from build123d import *

# Parameters (mm, degrees)
F0_R        = 1.5875
F1_DEPTH    = 6.35
F2_R        = 10.795
F4_R        = 19.05
F6_T        = 3.175
F6_T3_DEPTH = 12.7
F7_R        = 6.477
F8_DEPTH    = 19.051
F9_R        = 5.08


# Not quite as in the source:
# - two fillets or chamfers of one size are made in one step
# - a shell that OpenCascade refuses in one call is made with other operations: the cavity is built on its own and cut out


with BuildPart() as f1:
    # F0 (on Front) → F1 (new body)
    with BuildSketch(Plane.XZ):
        with BuildLine():
            ThreePointArc((35.2153805779, 11.4421707601), (39.8917386836, 9.0594472943), (42.2744621493, 13.7358054))
            ThreePointArc((42.2744621493, 13.7358054), (0, 44.45), (-42.2744621493, 13.7358054))
            ThreePointArc((-42.2744621493, 13.7358054), (-39.8917386836, 9.0594472943), (-35.2153805779, 11.4421707601))
            ThreePointArc((-35.2153805779, 11.4421707601), (-18.0952762982, 14.4949657749), (-6.0392088785, 1.9622579143))
            ThreePointArc((-6.0392088785, 1.9622579143), (0, -6.35), (6.0392088785, 1.9622579143))
            ThreePointArc((6.0392088785, 1.9622579143), (18.0952762982, 14.4949657749), (35.2153805779, 11.4421707601))
        make_face()
        Circle(F0_R, mode=Mode.SUBTRACT)
        with Locations((-39.2548577101, 12.7546764428)):
            Circle(F0_R, mode=Mode.SUBTRACT)
        with Locations((39.2548577101, 12.7546764428)):
            Circle(F0_R, mode=Mode.SUBTRACT)
        with Locations((-12.7546764428, 39.2548577101)):
            Circle(F0_R, mode=Mode.SUBTRACT)
        with Locations((12.7546764428, 39.2548577101)):
            Circle(F0_R, mode=Mode.SUBTRACT)
    extrude(amount=F1_DEPTH)

    # F2 (on face) → F5 section 0
    with BuildSketch(Plane.XZ.offset(6.35)):
        with Locations((0, 28.575)):
            Circle(F2_R)
    # F4 (on offset) → F5 section 1
    with BuildSketch(Plane.XZ.offset(19.05)):
        with Locations((0, 28.575)):
            Circle(F4_R)
    loft()

    # F6: shell of thickness 3.175, made by hand


with BuildPart() as f6_core1:
    # F6_t2: copy of F1
    add(f1.part)

    # the walls: a layer under each face that stays
    f6_faces = [f6_core1.faces().sort_by_distance(p)[0] for p in [
        (18.0952762982, -3.175, 14.4949657749),
        (0, -3.175, -6.35),
        (39.8917386836, -3.175, 9.0594472943),
        (0, 0, 19.05),
        (-28.3040667791, -6.35, 19.05),
        (-18.0952762982, -3.175, 14.4949657749),
        (0, -3.175, 44.45),
        (-39.8917386836, -3.175, 9.0594472943),
        (-1.5875, -3.175, 0),
        (-40.8423577101, -3.175, 12.7546764428),
        (37.6673577101, -3.175, 12.7546764428),
        (-14.3421764428, -3.175, 39.2548577101),
        (11.1671764428, -3.175, 39.2548577101),
        (-14.9225, -12.7, 28.575),
    ]]
    thicken(f6_faces, amount=-F6_T, mode=Mode.SUBTRACT)

    # F6_s4 → F6_t3 (cut)
    with BuildSketch(Plane.XZ.offset(-3.175)):
        Polygon((6.0999585135, 1.9634355139), (2.9838498192, 2.8256269079), (2.7217112336, 1.8979499721), (3.0196044392, 0.9811289571), align=None)
        Polygon((35.1655409151, 11.4074157187), (37.179742419, 13.9365459438), (37.9370918115, 13.3401207322), (38.2349850172, 12.4232997172), align=None)
        Polygon((-6.0999585135, 1.9634355139), (-3.0196044392, 0.9811289571), (-2.7217112336, 1.8979499721), (-2.9838498192, 2.8256269079), align=None)
        Polygon((-35.1655409151, 11.4074157187), (-37.179742419, 13.9365459438), (-37.9370918115, 13.3401207322), (-38.2349850172, 12.4232997172), align=None)
    extrude(amount=F6_T3_DEPTH, mode=Mode.SUBTRACT)

    # F6_s5 → F6_t6 (revolve, cut)
    with BuildSketch(Plane.XY.offset(28.575)):
        Polygon((10.8216205848, -6.3644466199), (10.795, -3.175), (4.9444718097, -3.175), (8.1329415182, -8.0803380131), align=None)
    revolve(axis=Axis((0, -6.35, 28.575), (0, -1, 0)), mode=Mode.SUBTRACT)


with BuildPart() as f1_1:
    add(f1.part)

    # what is left inside the walls is the cavity
    f6_cavity = [f6_core1.part.solids().sort_by_distance(p)[0] for p in [
        (-10.483081, -11.754195, 28.575),
    ]]
    add(f6_cavity, mode=Mode.SUBTRACT)

    # F7 (on face) → F8 (cut, through all)
    with BuildSketch(Plane.XZ.offset(19.05)):
        with Locations((0, 28.575)):
            Circle(F7_R)
    extrude(amount=-F8_DEPTH, mode=Mode.SUBTRACT)

    # F9
    f9_edges = [f1_1.edges().sort_by_distance(p)[0] for p in [
        (6.039209, -3.175, 1.962258),
        (-6.039209, -3.175, 1.962258),
        (-15.263222, -19.05, 28.575),
    ]]
    fillet(f9_edges, radius=F9_R)


solid = f1_1.part
Check sheet for the modelled part. Datum: model origin and axes. Units: mm. A direction names the side the tool comes from. Round coordinates to 2 decimals unless told otherwise and drop trailing zeros. Order: outer loops, then holes, each group sorted by start corner. A loop starts at its lowest first (then second) coordinate and runs counter-clockwise, first axis right, second up.
(1) Draft check along Z on faces 4 (the flat face through (9, -6.35, 19)), 5 (the cylindrical face through (-13.099, -3.131, 37.705)), 6 (the cylindrical face through (12.411, -3.131, 37.705)), 7 (the cylindrical face through (18.648, -3.131, 14.665)). Enter one of: pulls with the +Z half, pulls with the -Z half, needs draft (parallel to the pull), parting line crosses it, or undercut.
(2) Cross-section at C-C, the plane x = -25.5. Enter the section's corners in (y, z).
(3) Scan lines: probe 1 along Y at (x, z) = (26, 29); probe 2 along Y at (x, z) = (-11, 23); probe 3 along X at (y, z) = (-13.25, 34). Record each from-to range of solid material in increasing order.
(4) Cross-section at A-A, the plane z = 0. Enter the section's corners in (x, y).
(5) Go/stop test with flat-tipped pins: P1, Ø1.9, axis at x = -39.25, z = 12.75, coming from the -Y side; P2, Ø5, axis at x = 11, y = -16, coming from the +Z side; P3, Ø2, axis at x = 9.5, y = -2.5, coming from the -Z side; P4, Ø3, axis at x = 12.75, z = 39.25, coming from the +Y side. Record where each tip stops, or that it passes through.
(6) Access from +Z, -Z, +X, -X, +Y, -Y to the whole of each face (thin tool, end or side, straight path). Record for faces 1 (the conical face through (-1.473, -7.144, 39.79)), 2 (the cylindrical face through (0.782, -3.131, 44.443)), 3 (the flat face through (-1, 0, 19)).
(7) Cross-section at B-B, the plane y = -12. Enter the section's corners in (x, z) (1 decimal), and give its area (3 significant figures).
Check sheet entries:
1. face 4: needs draft
1. face 5: undercut
1. face 6: undercut
1. face 7: pulls with the -Z half
2. outline: (-6.35, 15.32) - (0, 15.32) - (0, 36.41) - (-6.35, 36.41) - close
3. probe 1: y = -6.35 to 0
3. probe 2: y = -14.54 to -8.71, -6.35 to 0
3. probe 3: x = -14.28 to -10.13, 10.13 to 14.28
4. outline: (-6.35, -6.35) - (-1.59, -6.35) - (-1.59, 0) - (-6.35, 0) - close; (1.59, -6.35) - (6.35, -6.35) - (6.35, 0) - (1.59, 0) - close
5. P1: passes through
5. P2: stops at z = 44.3
5. P3: stops at z = 7.27
5. P4: stops at y = -13.02
6. face 1: none
6. face 2: +Z, +Y
6. face 3: +Z, -Z, +X, -X, +Y
7. outline: circle Ø28.9 at (0, 28.6); hole circle Ø21.4 at (0, 28.6)
7. area: 299 mm2
